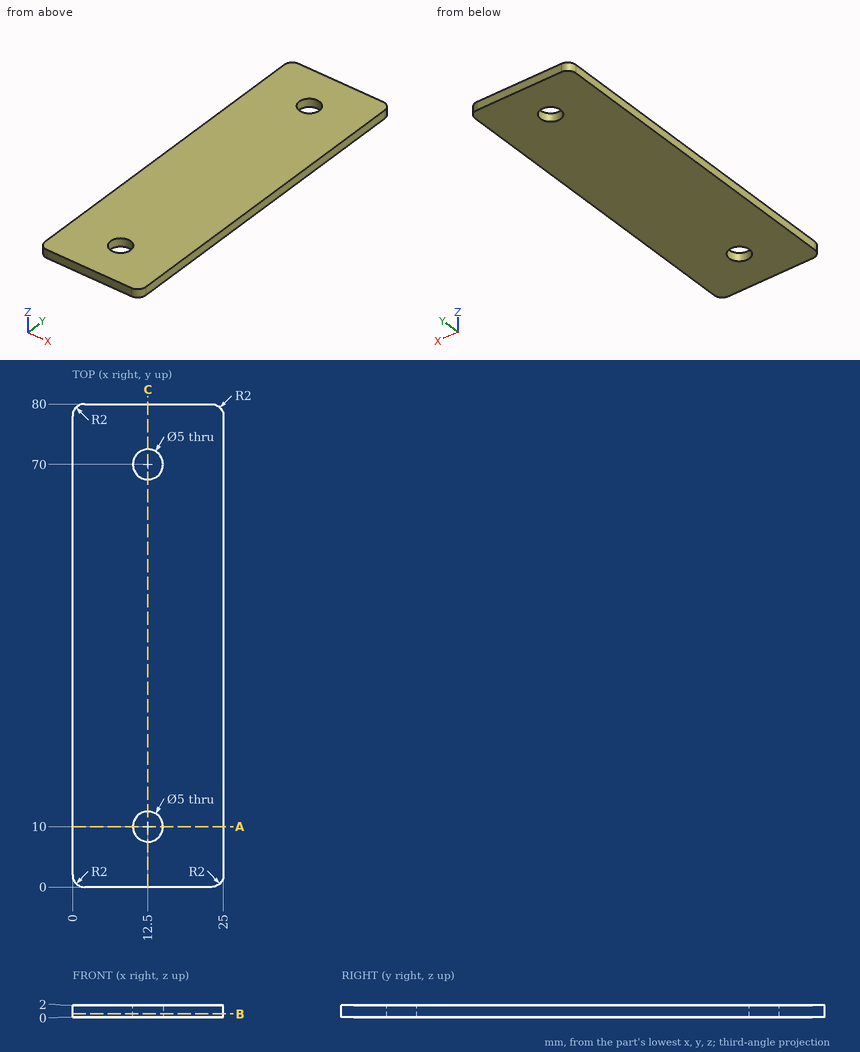
Source: three-view drawing plus pictorial views. Frame: mm from the lowest corner of the part. Coordinates: 2 decimals unless noted, no trailing zeros. Loops run counter-clockwise (first coordinate to the right, second up) from the corner with the lowest first, then second, coordinate; pieces in that order, holes last. Notation, with made-up numbers: (-1, 16.25) -> (6, 16.25) arc R5 cw to (6, 24.25) -> close; hole circle Ø11 at (64, 39.25). An arc over 180 degrees is marked (long way). Write each question's results on one line, items separated by ' | '. Start each with the question number.
Q1. Section C-C, the plane x = 12.5. Return the cut outline in (y, z).
Q2. Ray query, line 1 (Y direction, x = 12.5, z = 1); line 2 (Y direction, x = 10.5, z = 0.2); line 3 (X direction, y = 11.5, z = 0.3). Return the intervals inside material, ascending. Write a range as from..to.
Q3. Section B-B, the plane z = 0.55. Return the cut outline in (x, y), plus the area to 3 significant figures.
Q4. Section A-A, the plane y = 10. Return the cut outline in (x, z), plus the area to 3 significant figures.
Found:
1) outline: (0, 0) -> (7.5, 0) -> (7.5, 2) -> (0, 2) -> close; (12.5, 0) -> (67.5, 0) -> (67.5, 2) -> (12.5, 2) -> close; (72.5, 0) -> (80, 0) -> (80, 2) -> (72.5, 2) -> close
2) line 1: 0..7.5, 12.5..67.5, 72.5..80 | line 2: 0..8.5, 11.5..68.5, 71.5..80 | line 3: 0..10.5, 14.5..25
3) outline: (0, 2) arc R2 ccw to (2, 0) -> (23, 0) arc R2 ccw to (25, 2) -> (25, 78) arc R2 ccw to (23, 80) -> (2, 80) arc R2 ccw to (0, 78) -> close; hole circle Ø5 at (12.5, 10); hole circle Ø5 at (12.5, 70) | area: 1,960 mm2
4) outline: (0, 0) -> (10, 0) -> (10, 2) -> (0, 2) -> close; (15, 0) -> (25, 0) -> (25, 2) -> (15, 2) -> close | area: 40.0 mm2
